```python
from build123d import *

# Parameters (mm, degrees)
F0_R      = 48.895
F1_DEPTH  = 22.86
F3_DEPTH  = 22.861
F5_R      = 46.99
F6_DEPTH  = 12.7
F7_R      = 44.45
F8_DEPTH  = 21.59
F9_W      = 4.445
F9_H      = 3.048
F10_DEPTH = 48.896
F11_SIZE  = 1.27
F12_R     = 0.635
F13_DEPTH = 48.896


with BuildPart() as f1:
    # F0 (on Top) → F1 (new body)
    with BuildSketch(Plane.XY):
        Circle(F0_R)
    extrude(amount=-F1_DEPTH)

    # F2 (on Top) → F3 (cut, through all)
    with BuildSketch(Plane.XY):
        with BuildLine():
            Line((-2.6737949155, -21.209), (2.6737949155, -21.209))
            ThreePointArc((2.6737949155, -21.209), (6.5405, -15.24), (2.6737949155, -9.271))
            Line((2.6737949155, -9.271), (-2.6737949155, -9.271))
            ThreePointArc((-2.6737949155, -9.271), (-6.5405, -15.24), (-2.6737949155, -21.209))
        make_face()
    extrude(amount=-F3_DEPTH, mode=Mode.SUBTRACT)

    # F5 (on offset) → F6 (cut)
    with BuildSketch(Plane(origin=(0, 0, -22.86), x_dir=(1, 0, 0), z_dir=(0, 0, -1))):
        Circle(F5_R)
    extrude(amount=-F6_DEPTH, mode=Mode.SUBTRACT)

    # F7 (on offset) → F8 (cut)
    with BuildSketch(Plane(origin=(0, 0, -22.86), x_dir=(1, 0, 0), z_dir=(0, 0, -1))):
        Circle(F7_R)
    extrude(amount=-F8_DEPTH, mode=Mode.SUBTRACT)

    # F9 (on Right) → F10 (cut, through all)
    with BuildSketch(Plane.YZ):
        with Locations((-15.24, -21.336)):
            Rectangle(F9_W, F9_H)
    extrude(amount=F10_DEPTH, mode=Mode.SUBTRACT)

    # F11
    f11_edges = [f1.edges().sort_by_distance(p)[0] for p in [
        (44.44345, -15.259091, -19.812),
    ]]
    chamfer(f11_edges, length=F11_SIZE)

    # F12 (on Front) → F13 (cut, through all)
    with BuildSketch(Plane.XZ):
        with Locations((0, -16.002)):
            Circle(F12_R)
    extrude(amount=-F13_DEPTH, mode=Mode.SUBTRACT)


solid = f1.part
```
Could you check a few things on this model? Use its own coordinates, in mm. A direction names the side the tool comes from. Coordinates: 2 decimals unless noted, no trailing zeros. Order: outer loops, then holes, each group sorted by start corner. A loop starts at its lowest first (then second) coordinate and runs counter-clockwise, first axis right, second up. Notation, with made-up numbers: M -10,66.25 L 8,66.25 A30 ccw 8,91.25 Z; hole C -38.75,35 d3. An arc over 180 degrees is marked long. Use one line per item in the form item = value. Start each with the question number.
1. Suppose I cut it at D-D on x = 35.5. Write out the boundary of the cut face in (y, z).
2. Suppose I cut it at C-C on y = -20. Write out the boundary of the cut face in (x, z), then the cut area to 3 significant figures.
3. Suppose I cut it at A-A on y = 0. Write out the boundary of the cut face in (x, z) (3 decimals), then the cut area to 3 significant figures.
4. We'd pull the mould along Y, two halves only. Please class faces 5 (the conical face through (45.105, -15.258, -19.168)), 6 (the cylindrical face through (-10.599, -47.732, -11.27)), 7 (the flat face through (-1, 1, 0)), 8 (the cylindrical face through (42.397, -13.352, -5.777)): +Y half, -Y half, draft (parallel to the pull), parting line (faces both ways), or undercut.
5. For pin 1 (3 mm diameter, centred on x = -37, z = -14, fed in from -Y); pin 2 (8 mm diameter, centred on x = 21, z = -15.5, fed in from +Y); pin 3 (5 mm diameter, centred on x = -34, z = -17, fed in from -Y), each with a flat end and sliding along its axis, tell me the tip position at first contact or that it passes through.
6. On a 3-axis mill with a long thin cutter (end or side, diameter ignored), from which of +Z, -Z, +X, -X, +Y, -Y can I reach the whole of each face in a straight line? I mean faces 1 (the flat face through (-26, 40, -22.86)), 2 (the cylindrical face through (-6.54, -15.13, -0.63)), 3 (the flat face through (46.1, -15.3, -19.812)), 4 (the flat face through (-28, 35, -10.16)). Say none if no direction works.
7. Please list where these lines run through material, in increasing order: line 1 (X direction, y = 0, z = -5) (3 decimals); line 2 (X direction, y = 0, z = -17.5) (3 decimals).
8. Suppose I cut it at B-B on x = -4. Write out the boundary of the cut face in (y, z), then the cut area to 3 significant figures.
Geometry says:
q1.outline = M -33.62,-22.86 L -30.79,-22.86 L -30.79,-10.16 L -26.75,-10.16 L -26.75,-1.27 L 26.75,-1.27 L 26.75,-10.16 L 30.79,-10.16 L 30.79,-22.86 L 33.62,-22.86 L 33.62,0 L -33.62,0 Z
q2.outline = M -44.62,-22.86 L -42.52,-22.86 L -42.52,-10.16 L -39.7,-10.16 L -39.7,-1.27 L -4.49,-1.27 L -4.49,0 L -44.62,0 Z; M 4.49,-1.27 L 39.7,-1.27 L 39.7,-10.16 L 42.52,-10.16 L 42.52,-22.86 L 44.62,-22.86 L 44.62,0 L 4.49,0 Z
q2.area = 243 mm^2
q3.outline = M -48.895,-22.86 L -46.99,-22.86 L -46.99,-10.16 L -44.45,-10.16 L -44.45,-1.27 L 44.45,-1.27 L 44.45,-10.16 L 46.99,-10.16 L 46.99,-22.86 L 48.895,-22.86 L 48.895,0 L -48.895,0 Z
q3.area = 252 mm^2
q4.face_5 = undercut
q4.face_6 = parting line
q4.face_7 = draft
q4.face_8 = undercut
q5.pin_1 = -33.62
q5.pin_2 = 45.84
q5.pin_3 = -37.4
q6.face_1 = -Z, +X, -X, +Y, -Y
q6.face_2 = +Z, -Z
q6.face_3 = -Z, +X
q6.face_4 = -Z
q7.line_1 = -48.895 to -44.45, 44.45 to 48.895
q7.line_2 = -48.895 to -46.99, 46.99 to 48.895
q8.outline = M -48.73,-22.86 L -46.82,-22.86 L -46.82,-10.16 L -44.27,-10.16 L -44.27,-1.27 L -20.41,-1.27 L -20.41,0 L -48.73,0 Z; M -10.07,-1.27 L 44.27,-1.27 L 44.27,-10.16 L 46.82,-10.16 L 46.82,-22.86 L 48.73,-22.86 L 48.73,0 L -10.07,0 Z
q8.area = 239 mm^2
